```python
from build123d import *

# Parameters (mm, degrees)
SKETCH1_W           = 100
SKETCH1_H           = 100
BOSS_EXTRUDE1_DEPTH = 10
CUT_EXTRUDE1_DEPTH  = 72.414284285
SKETCH3_W           = 75
SKETCH3_H           = 75
CUT_EXTRUDE2_DEPTH  = 10
BOSS_EXTRUDE2_DEPTH = 10
SKETCH10_R          = 1
CUT_EXTRUDE7_DEPTH  = 72.414284285
SKETCH11_R          = 1
CUT_EXTRUDE8_DEPTH  = 72.414284285
SKETCH12_R          = 1
CUT_EXTRUDE9_DEPTH  = 72.414284285
SKETCH9_R           = 1
CUT_EXTRUDE11_DEPTH = 10
SKETCH13_R          = 1
CUT_EXTRUDE12_DEPTH = 10
SKETCH14_R          = 1
CUT_EXTRUDE13_DEPTH = 10
SKETCH15_R          = 1
CUT_EXTRUDE14_DEPTH = 10
SKETCH16_R          = 1
CUT_EXTRUDE15_DEPTH = 10
SKETCH17_R          = 1
CUT_EXTRUDE16_DEPTH = 10
SKETCH18_R          = 1
CUT_EXTRUDE17_DEPTH = 10
SKETCH19_R          = 1
CUT_EXTRUDE18_DEPTH = 10


with BuildPart() as part:
    # Sketch1 → Boss-Extrude1 (new body)
    with BuildSketch(Plane(origin=(0, 0, 0), x_dir=(1, 0, 0), z_dir=(0, 1, 0))):
        Rectangle(SKETCH1_W, SKETCH1_H)
    extrude(amount=BOSS_EXTRUDE1_DEPTH)

    # Sketch2 → Cut-Extrude1 (cut, through all)
    with BuildSketch(Plane(origin=(0, 10, 0), x_dir=(1, 0, 0), z_dir=(0, 1, 0))):
        Polygon((35, 50), (35, 45), (45, 45), (45, 35), (50, 35), (50, 50), align=None)
        Polygon((-45, 35), (-50, 35), (-50, 50), (-35, 50), (-35, 45), (-45, 45), align=None)
        Polygon((-45, -35), (-50, -35), (-50, -50), (-35, -50), (-35, -45), (-45, -45), align=None)
        Polygon((35, -50), (35, -45), (45, -45), (45, -35), (50, -35), (50, -50), align=None)
    extrude(amount=-CUT_EXTRUDE1_DEPTH, mode=Mode.SUBTRACT)

    # Sketch3 → Cut-Extrude2 (cut)
    with BuildSketch(Plane(origin=(0, 10, 0), x_dir=(1, 0, 0), z_dir=(0, 1, 0))):
        Rectangle(SKETCH3_W, SKETCH3_H)
    extrude(amount=-CUT_EXTRUDE2_DEPTH, mode=Mode.SUBTRACT)

    # Sketch4 → Boss-Extrude2 (add)
    with BuildSketch(Plane(origin=(0, 10, 0), x_dir=(1, 0, 0), z_dir=(0, 1, 0))):
        Polygon((45.985281374, 0), (0, 45.985281374), (-45.985281374, 0), (0, -45.985281374), align=None)
        Polygon((0, 37.5), (-37.5, 0), (0, -37.5), (37.5, 0), align=None, mode=Mode.SUBTRACT)
    extrude(amount=-BOSS_EXTRUDE2_DEPTH)

    # Sketch10 → Cut-Extrude7 (cut, through all)
    with BuildSketch(Plane(origin=(0, 10, 0), x_dir=(1, 0, 0), z_dir=(0, 1, 0))):
        with Locations(Location((0, 47, 0), (0, 0, 270))):
            Circle(SKETCH10_R)
        with Locations(Location((0, -47, 0), (0, 0, 90))):
            Circle(SKETCH10_R)
    extrude(amount=-CUT_EXTRUDE7_DEPTH, mode=Mode.SUBTRACT)

    # Sketch11 → Cut-Extrude8 (cut, through all)
    with BuildSketch(Plane(origin=(0, 10, 0), x_dir=(1, 0, 0), z_dir=(0, 1, 0))):
        with Locations(Location((-47, 0, 0), (0, 0, 270))):
            Circle(SKETCH11_R)
        with Locations(Location((47, 0, 0), (0, 0, 90))):
            Circle(SKETCH11_R)
    extrude(amount=-CUT_EXTRUDE8_DEPTH, mode=Mode.SUBTRACT)

    # Sketch12 → Cut-Extrude9 (cut, through all)
    with BuildSketch(Plane(origin=(0, 10, 0), x_dir=(1, 0, 0), z_dir=(0, 1, 0))):
        with Locations(Location((-20.871320344, 20.871320344, 0), (0, 0, 270))):
            Circle(SKETCH12_R)
        with Locations(Location((20.871320344, 20.871320344, 0), (0, 0, 90))):
            Circle(SKETCH12_R)
        with Locations(Location((20.871320344, -20.871320344, 0), (0, 0, 270))):
            Circle(SKETCH12_R)
        with Locations(Location((-20.871320344, -20.871320344, 0), (0, 0, 90))):
            Circle(SKETCH12_R)
    extrude(amount=-CUT_EXTRUDE9_DEPTH, mode=Mode.SUBTRACT)

    # Sketch9 → Cut-Extrude11 (cut)
    with BuildSketch(Plane.ZY.offset(45)):
        with Locations((-40, 3)):
            Circle(SKETCH9_R)
    extrude(amount=-CUT_EXTRUDE11_DEPTH, mode=Mode.SUBTRACT)

    # Sketch13 → Cut-Extrude12 (cut)
    with BuildSketch(Plane(origin=(0, 0, -45), x_dir=(-1, 0, 0), z_dir=(0, 0, -1))):
        with Locations((40, 7)):
            Circle(SKETCH13_R)
    extrude(amount=-CUT_EXTRUDE12_DEPTH, mode=Mode.SUBTRACT)

    # Sketch14 → Cut-Extrude13 (cut)
    with BuildSketch(Plane.ZY.offset(45)):
        with Locations((40, 7)):
            Circle(SKETCH14_R)
    extrude(amount=-CUT_EXTRUDE13_DEPTH, mode=Mode.SUBTRACT)

    # Sketch15 → Cut-Extrude14 (cut)
    with BuildSketch(Plane.XY.offset(45)):
        with Locations((-40, 3)):
            Circle(SKETCH15_R)
    extrude(amount=-CUT_EXTRUDE14_DEPTH, mode=Mode.SUBTRACT)

    # Sketch16 → Cut-Extrude15 (cut)
    with BuildSketch(Plane.XY.offset(45)):
        with Locations((40, 7)):
            Circle(SKETCH16_R)
    extrude(amount=-CUT_EXTRUDE15_DEPTH, mode=Mode.SUBTRACT)

    # Sketch17 → Cut-Extrude16 (cut)
    with BuildSketch(Plane(origin=(45, 0, 0), x_dir=(0, 0, -1), z_dir=(1, 0, 0))):
        with Locations((-40, 3)):
            Circle(SKETCH17_R)
    extrude(amount=-CUT_EXTRUDE16_DEPTH, mode=Mode.SUBTRACT)

    # Sketch18 → Cut-Extrude17 (cut)
    with BuildSketch(Plane(origin=(45, 0, 0), x_dir=(0, 0, -1), z_dir=(1, 0, 0))):
        with Locations((40, 7)):
            Circle(SKETCH18_R)
    extrude(amount=-CUT_EXTRUDE17_DEPTH, mode=Mode.SUBTRACT)

    # Sketch19 → Cut-Extrude18 (cut)
    with BuildSketch(Plane(origin=(0, 0, -45), x_dir=(-1, 0, 0), z_dir=(0, 0, -1))):
        with Locations((-40, 3)):
            Circle(SKETCH19_R)
    extrude(amount=-CUT_EXTRUDE18_DEPTH, mode=Mode.SUBTRACT)


solid = part.part
```
The listing builds one solid part. Answer for the finished solid, in the listing's coordinates (mm). A direction names the side the tool comes from. Coordinates: 2 decimals unless noted, no trailing zeros. Write each loop counter-clockwise with the first axis right and the second up, starting at its lowest first coordinate (ties: lowest second). Pieces come first, ordered by that corner, then holes. Notation, with made-up numbers: (67, -23) - (112, -23) arc R11 ccw to (112, -7) - close; hole circle Ø7 at (49.5, 35). An arc over 180 degrees is marked (long way). Return JSON: item names as keys, results as strings. Group by question number.
Q1. The part is cut by section B-B on z = -15.5. Write down the section's boundary in (x, y), and give its area (3 significant figures).
Q2. The part is cut by section A-A on x = -6. Write down the section's boundary in (y, z), and give its area (3 significant figures).
Q3. Which of the six approach directions +Z, -Z, +X, -X, +Y, -Y give full straight-line access (tool end or side, diameter ignored) to faces 1 (the flat face through (47, 5, 35)), 2 (the flat face through (-45, 5, 40)), 3 (the flat face through (-19, 5.1, 18.5)), 4 (the flat face through (-47, 5, -35)), 5 (the flat face through (35, 5, -48))?
Q4. For a pull along X with two mould halves and no side action, classify faces 6 (the flat face through (23.196, 5.07, -22.79)), 7 (the flat face through (-40, 5, 45)), 8 (the flat face through (45, 5, -40)), 9 (the flat face through (-23, 5, -37.5)) as +X half, -X half, draft (parallel to the pull), parting line (faces both ways), or undercut.
Q5. Find the intervals of material crossed by line 1 along X through (y, z) = (7.75, 0); line 2 along Y through (x, z) = (-40, 38.5); line 3 along Z through (x, y) = (35.5, 2.75), in increasing order. Write a range as [from, to].
Q6. The part is cut by section C-C on x = 25. Write down the section's boundary in (y, z), and give its area (3 significant figures).
Q7. Flat-ended cylindrical pins translate along their axes: pin 1 Ø3 at (x, z) = (-20.87, -20.87) entering from -Y; pin 2 Ø2.5 at (x, y) = (-40, 3) entering from +Z; pin 3 Ø1.2 at (y, z) = (3, 40) entering from +X; pin 4 Ø2.5 at (x, y) = (47, 2.5) entering from +Z. Find the tip coordinate at first contact, or state that the pin passes through.
Evaluation:
{
 "1": {"outline": "(-50, 0) - (-37.5, 0) - (-37.5, 10) - (-50, 10) - close; (-30.49, 0) - (-22, 0) - (-22, 10) - (-30.49, 10) - close; (22, 0) - (30.49, 0) - (30.49, 10) - (22, 10) - close; (37.5, 0) - (50, 0) - (50, 10) - (37.5, 10) - close", "area": "420 mm2"},
 "2": {"outline": "(0, -50) - (10, -50) - (10, -31.5) - (0, -31.5) - close; (0, 31.5) - (10, 31.5) - (10, 50) - (0, 50) - close", "area": "370 mm2"},
 "3": {"face 1": "+Z, +X, +Y, -Y", "face 2": "+Z, -X, +Y, -Y", "face 3": "+Y, -Y", "face 4": "-Z, -X, +Y, -Y", "face 5": "-Z, +X, +Y, -Y"},
 "4": {"face 6": "undercut", "face 7": "draft", "face 8": "+X half", "face 9": "undercut"},
 "5": {"line 1": "x = [-50, -48], [-46, -37.5], [37.5, 46], [48, 50]", "line 2": "y = [0, 2], [4, 10]", "line 3": "z = [-45, -37.5], [-10.49, -2], [2, 10.49], [37.5, 39.03], [40.97, 45]"},
 "6": {"outline": "(0, -50) - (10, -50) - (10, -37.5) - (0, -37.5) - close; (0, -20.99) - (10, -20.99) - (10, -12.5) - (0, -12.5) - close; (0, 12.5) - (10, 12.5) - (10, 20.99) - (0, 20.99) - close; (0, 37.5) - (10, 37.5) - (10, 50) - (0, 50) - close", "area": "420 mm2"},
 "7": {"pin 1": "stops at y = 0", "pin 2": "stops at z = 45", "pin 3": "stops at x = 35", "pin 4": "stops at z = 35"}
}
